Input: dimensioned drawing with shaded views. Units: mm. Origin: part minimum x, y, z. A direction names the side the tool comes from. Give positions to 0.01 mm unless a question says otherwise; leave off trailing zeros. Loops run counter-clockwise (first coordinate to the right, second up) from the corner with the lowest first, then second, coordinate; pieces in that order, holes last.
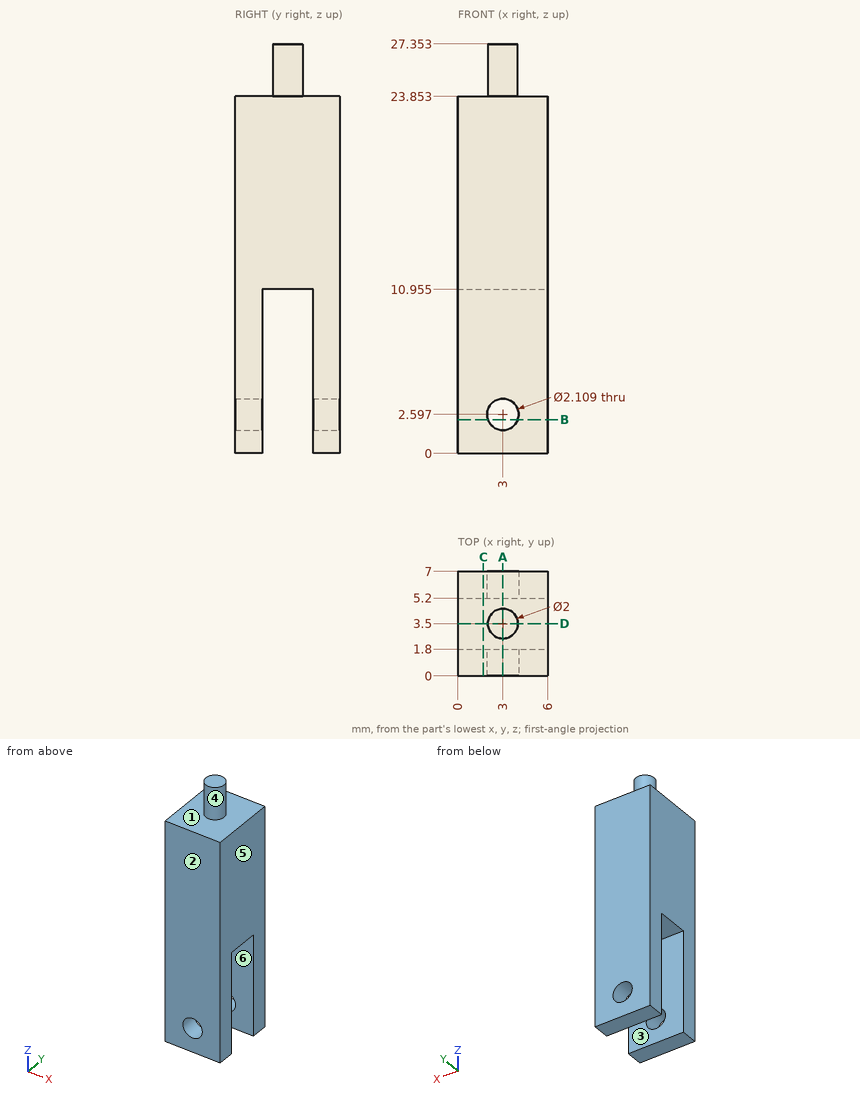
Item 1: Section query B-B on z = 2.25. Return loops of the section in (x, y) (1 decimal).
Values follow:
outline: (0, 0) - (2, 0) - (2, 1.8) - (0, 1.8) - close; (0, 5.2) - (2, 5.2) - (2, 7) - (0, 7) - close; (4, 0) - (6, 0) - (6, 1.8) - (4, 1.8) - close; (4, 5.2) - (6, 5.2) - (6, 7) - (4, 7) - close
Item 2: Pin query (flat end, axial travel): pin 1 (2 mm diameter, centred on x = 4, y = 1, fed in from +Z). Return the tip coordinate at first contact, or that it passes through.
Values follow:
pin 1: stops at z = 23.85
Item 3: Section query A-A on x = 3. Return loops of the section in (y, z) (1 decimal), plus the area to 3 significant figures.
Values follow:
outline: (0, 0) - (1.8, 0) - (1.8, 1.5) - (0, 1.5) - close; (0, 3.7) - (1.8, 3.7) - (1.8, 11) - (5.2, 11) - (5.2, 3.7) - (7, 3.7) - (7, 23.9) - (4.5, 23.9) - (4.5, 27.4) - (2.5, 27.4) - (2.5, 23.9) - (0, 23.9) - close; (5.2, 0) - (7, 0) - (7, 1.5) - (5.2, 1.5) - close
area: 129 mm2
Item 4: Ray query, probe 1 along Y at (x, z) = (1.5, 9.5); probe 2 along Z at (x, y) = (3, 0.4); probe 3 along Z at (x, y) = (5.3, 5.5). Return the intervals inside material, ascending.
Values follow:
probe 1: y = 0 to 1.8, 5.2 to 7
probe 2: z = 0 to 1.54, 3.65 to 23.85
probe 3: z = 0 to 23.85
Item 5: Section query D-D on y = 3.5. Return loops of the section in (x, z) (1 decimal).
Values follow:
outline: (0, 11) - (6, 11) - (6, 23.9) - (4, 23.9) - (4, 27.4) - (2, 27.4) - (2, 23.9) - (0, 23.9) - close
Item 6: Draft query along Y for the marked faces 1, 2 and 3. Return one class per face: +Y half, -Y half, draft (parallel to the pull), parting line (faces both ways), or undercut.
Values follow:
face 1: draft
face 2: -Y half
face 3: undercut
Item 7: Set-up query: the marked faces 4, 5 and 6. Return all of +Z, -Z, +X, -X, +Y, -Y with unobstructed straight access to the full face (end or side cutting, diameter ignored); none if empty.
Values follow:
face 4: +Z
face 5: +Z, -Z, +X, +Y, -Y
face 6: -Z, +X, -X
Item 8: Section query C-C on x = 1.7. Return loops of the section in (y, z) (1 decimal), plus the area to 3 significant figures.
Values follow:
outline: (0, 0) - (1.8, 0) - (1.8, 11) - (5.2, 11) - (5.2, 0) - (7, 0) - (7, 23.9) - (0, 23.9) - close
area: 130 mm2
